from build123d import *

# Parameters (mm, degrees)
BOSS_EXTRUDE1_DEPTH             = 20
SKETCH3_W                       = 3
SKETCH3_H                       = 20
BOSS_EXTRUDE3_DEPTH             = 31
BOSS_EXTRUDE3_DIRECTION_2_REACH = 77.374
SKETCH4_W                       = 3
SKETCH4_H                       = 10
BOSS_EXTRUDE4_DEPTH             = 15
SKETCH6_R                       = 2
CUT_EXTRUDE2_DEPTH              = 3


with BuildPart() as part:
    # Sketch1 → Boss-Extrude1 (new body)
    with BuildSketch(Plane.XY):
        with BuildLine():
            Line((0, -29.5), (0, -32.5))
            ThreePointArc((0, -32.5), (-32.4258356, -2.194353132), (-4.378691316, 32.203680882))
            Line((-4.378691316, 32.203680882), (-4.378691316, 29.173225093))
            ThreePointArc((-4.378691316, 29.173225093), (-29.418192843, -2.195433869), (0, -29.5))
        make_face()
    extrude(amount=BOSS_EXTRUDE1_DEPTH)

    # Sketch3 → Boss-Extrude3 (add)
    with BuildSketch(Plane(origin=(0, 32.5, 0), x_dir=(1, 0, 0), z_dir=(0, 1, 0))):
        with Locations((-5.878691316, -10)):
            Rectangle(SKETCH3_W, SKETCH3_H)
    extrude(amount=BOSS_EXTRUDE3_DEPTH)

    # Sketch3 → Boss-Extrude3 direction 2 (add, up to next)
    with BuildSketch(Plane(origin=(0, 32.5, 0), x_dir=(1, 0, 0), z_dir=(0, 1, 0)), mode=Mode.PRIVATE) as boss_extrude3_direction_2_sk1:
        with Locations((-5.878691316, -10)):
            Rectangle(SKETCH3_W, SKETCH3_H)
    boss_extrude3_direction_2_tool1 = extrude(boss_extrude3_direction_2_sk1.sketch, amount=-BOSS_EXTRUDE3_DIRECTION_2_REACH, mode=Mode.PRIVATE) - part.part
    add(boss_extrude3_direction_2_tool1.solids().sort_by_distance((-5.878691, 32.5, 10))[0])

    # Sketch4 → Boss-Extrude4 (add)
    with BuildSketch(Plane.ZY.offset(7.378691316)):
        with Locations((1.5, 58.5)):
            Rectangle(SKETCH4_W, SKETCH4_H)
    extrude(amount=BOSS_EXTRUDE4_DEPTH)

    # Sketch6 → Cut-Extrude2 (cut)
    with BuildSketch(Plane.XY.offset(3)):
        with Locations((-14.878691316, 58.5)):
            Circle(SKETCH6_R)
    extrude(amount=-CUT_EXTRUDE2_DEPTH, mode=Mode.SUBTRACT)


solid = part.part
Read the model definition and answer for the solid it produces. Units are mm, in the model's axes. A direction names the side the tool comes from. Give positions to 0.01 mm unless a question says otherwise; leave off trailing zeros. Write each loop counter-clockwise with the first axis right and the second up, starting at its lowest first coordinate (ties: lowest second). Pieces come first, ordered by that corner, then holes. Notation, with made-up numbers: M 22,-37.5 L 69,-37.5 A7 ccw 69,-26.5 Z; hole C 31,-0.75 d10. An arc over 180 degrees is marked long. One line per item, written item: value. Start each with the question number.
(1) Find section C-C (y = -3). Determine the outline of the cut face in (x, z).
(2) Find section A-A (y = 58.5). Determine the outline of the cut face in (x, z).
(3) A tool of negligible diameter and unlimited length cuts with its end or side. For faces 1 (the flat face through (-13, 57, 3)), 2 (the flat face through (-22.379, 59, 1)), 3 (the flat face through (-4.379, 47, 10)), 4 (the flat face through (-15, 53.5, 1)), from which of +Z, -Z, +X, -X, +Y, -Y can it reach the whole face along a straight path? Write none if from no direction.
(4) Find the intervals of material crossed by line 1 (Y direction, x = -16, z = 14.5); line 2 (X direction, y = 48, z = 6.75); line 3 (Y direction, x = -19, z = 15.75), in increasing order.
(5) Find section B-B (z = 16.75). Determine the outline of the cut face in (x, y).
(6) Find section D-D (y = 9). Determine the outline of the cut face in (x, z).
(7) Flat-ended cylindrical pins translate along their axes: pin 1 Ø5 at (x, z) = (-7, 2.5) entering from -Y; pin 2 Ø10 at (y, z) = (48.5, 10.5) entering from +X; pin 3 Ø3.5 at (y, z) = (59.5, 1.5) entering from -X; pin 4 Ø3.5 at (x, y) = (-14.88, 58.5) entering from -Z. Find the tip coordinate at first contact, or state that the pin passes through.
(8) Determine the mould class of faces 5 (the flat face through (-7, 63.5, 6)), 6 (the cylindrical face through (-15.139, 60.483, 1.521)), 7 (the flat face through (-17, 26, 0)) for opening direction Y: pulls with the +Y half, pulls with the -Y half, needs draft (parallel to the pull), parting line crosses it, or undercut.
Results below:
1. outline: M -32.36,0 L -29.35,0 L -29.35,20 L -32.36,20 Z
2. outline: M -22.38,0 L -16.88,0 L -16.88,3 L -22.38,3 Z; M -12.88,0 L -4.38,0 L -4.38,20 L -7.38,20 L -7.38,3 L -12.88,3 Z
3. face 1: +Z, -X, +Y
3. face 2: +Z, -Z, -X, +Y
3. face 3: +Z, -Z, +X, +Y
3. face 4: +Z, -Z, -X
4. line 1: y = -28.29 to -24.78, 24.78 to 28.29
4. line 2: x = -7.38 to -4.38
4. line 3: y = -26.37 to -22.57, 22.57 to 26.37
5. outline: M -7.38,31.65 A32.5 ccw 0,-32.5 L 0,-29.5 A29.5 cw -4.38,29.17 L -4.38,63.5 L -7.38,63.5 Z
6. outline: M -31.23,0 L -28.09,0 L -28.09,20 L -31.23,20 Z
7. pin 1: stops at y = -32.19
7. pin 2: stops at x = -4.38
7. pin 3: stops at x = -22.38
7. pin 4: passes through
8. face 5: pulls with the +Y half
8. face 6: undercut
8. face 7: needs draft
